```python
from build123d import *

# Parameters (mm, degrees)
BOSS_EXTRUDE1_DEPTH = 18
SKETCH6_W           = 70
SKETCH6_H           = 36
SKETCH6_R           = 2.5
BOSS_EXTRUDE2_DEPTH = 5
SKETCH7_R           = 10
CUT_EXTRUDE1_DEPTH  = 19
SKETCH8_R           = 14.2875
CUT_EXTRUDE2_DEPTH  = 6.35
CHAMFER1_SIZE       = 0.5
BOSS_EXTRUDE3_DEPTH = 6.35
BOSS_EXTRUDE4_DEPTH = 6.35


with BuildPart() as part:
    # Sketch3 → Boss-Extrude1 (new body)
    with BuildSketch(Plane.XY):
        with BuildLine():
            Line((-20, 0), (-20, -40))
            Line((-20, -40), (20, -40))
            Line((20, -40), (20, 0))
            ThreePointArc((20, 0), (0, 20), (-20, 0))
        make_face()
    extrude(amount=BOSS_EXTRUDE1_DEPTH)

    # Sketch6 → Boss-Extrude2 (add)
    with BuildSketch(Plane.XZ.offset(40)):
        Rectangle(SKETCH6_W, SKETCH6_H)
        with Locations((28, 0)):
            Circle(SKETCH6_R, mode=Mode.SUBTRACT)
        with Locations((-28, 0)):
            Circle(SKETCH6_R, mode=Mode.SUBTRACT)
    extrude(amount=BOSS_EXTRUDE2_DEPTH)

    # Sketch7 → Cut-Extrude1 (cut, through all)
    with BuildSketch(Plane(origin=(0, 0, 0), x_dir=(-1, 0, 0), z_dir=(0, 0, -1))):
        Circle(SKETCH7_R)
    extrude(amount=-CUT_EXTRUDE1_DEPTH, mode=Mode.SUBTRACT)

    # Sketch8 → Cut-Extrude2 (cut)
    with BuildSketch(Plane(origin=(0, 0, 0), x_dir=(-1, 0, 0), z_dir=(0, 0, -1))):
        Circle(SKETCH8_R)
    extrude(amount=-CUT_EXTRUDE2_DEPTH, mode=Mode.SUBTRACT)

    # Chamfer1
    chamfer1_edges = [part.edges().sort_by_distance(p)[0] for p in [
        (14.2875, 0, 0),
    ]]
    chamfer(chamfer1_edges, length=CHAMFER1_SIZE)

    # Sketch9 → Boss-Extrude3 (add)
    with BuildSketch(Plane(origin=(20, 0, 0), x_dir=(0, 0, -1), z_dir=(1, 0, 0))):
        Polygon((18, -40), (0, -10), (0, -40), align=None)
    boss_extrude3 = extrude(amount=-BOSS_EXTRUDE3_DEPTH)

    # Mirror1: Boss-Extrude3 across plane
    add(boss_extrude3.mirror(Plane(origin=(0, 0, 0), x_dir=(0, 0, 1), z_dir=(1, 0, 0))))

    # Sketch10 → Boss-Extrude4 (add)
    with BuildSketch(Plane.XY.offset(18)):
        Polygon((-20, -10), (-35, -40), (-20, -40), align=None)
        Polygon((20, -10), (20, -40), (35, -40), align=None)
    extrude(amount=-BOSS_EXTRUDE4_DEPTH)


solid = part.part
```
Geometry: final body of the model. Coordinates: model frame, mm. A direction names the side the tool comes from. Give positions to 0.01 mm unless a question says otherwise; leave off trailing zeros. Loops run counter-clockwise (first coordinate to the right, second up) from the corner with the lowest first, then second, coordinate; pieces in that order, holes last. Notation, with made-up numbers: (25, -18) -> (82, -18) arc R21 ccw to (82, -10) -> close; hole circle Ø10 at (-33, 12). An arc over 180 degrees is marked (long way). Return JSON: item names as keys, results as strings.
Item 1: Pin query (flat end, axial travel): P1, Ø6, axis at x = -28, z = 0, coming from the +Y side; P2, Ø3, axis at y = -25.5, z = 5, coming from the -X side; P3, Ø11, axis at y = -24, z = 1.5, coming from the +X side. Return the tip coordinate at first contact, or that it passes through.
Filled in:
{"P1": "y = -40", "P2": "x = -20", "P3": "x = 20"}
Item 2: Section B-B, the plane z = 10. Output: boundary loops of the cut face in (x, y), plus the area to 3 significant figures.
Filled in:
{"outline": "(-35, -45) -> (35, -45) -> (35, -40) -> (20, -40) -> (20, 0) arc R20 ccw to (-20, 0) -> (-20, -40) -> (-35, -40) -> close; hole circle Ø20 at (0, 0)", "area": "2,260 mm^2"}
Item 3: Section A-A, the plane x = 28. Output: boundary loops of the cut face in (y, z).
Filled in:
{"outline": "(-45, -18) -> (-40, -18) -> (-40, -2.5) -> (-45, -2.5) -> close; (-45, 2.5) -> (-40, 2.5) -> (-40, 11.65) -> (-26, 11.65) -> (-26, 18) -> (-45, 18) -> close"}
Item 4: Line query: line 1 (Y direction, x = 0, z = 9); line 2 (Y direction, x = 0, z = 1); line 3 (Y direction, x = 4, z = -5). Output: solid intervals per line, ascending.
Filled in:
{"line 1": "-45 to -10, 10 to 20", "line 2": "-45 to -14.29, 14.29 to 20", "line 3": "-45 to -40"}
Item 5: Section D-D, the plane x = -29.5. Output: boundary loops of the cut face in (y, z).
Filled in:
{"outline": "(-45, -18) -> (-40, -18) -> (-40, -2) -> (-45, -2) -> close; (-45, 2) -> (-40, 2) -> (-40, 11.65) -> (-29, 11.65) -> (-29, 18) -> (-45, 18) -> close"}
Item 6: Mould query, pull axis Y, two halves, no side actions, for faces 1 (the flat face through (27, -40, -3)), 2 (the cylindrical face through (14.274, 0.628, 3.384)), 3 (the flat face through (10, -3, 6.35)), 4 (the flat face through (-13.65, -31, -5)). Classes: released by +Y, released by -Y, zero draft, split by the parting line, or undercut.
Filled in:
{"face 1": "released by +Y", "face 2": "undercut", "face 3": "undercut", "face 4": "zero draft"}
Item 7: Section C-C, the plane y = -21. Output: boundary loops of the cut face in (x, z).
Filled in:
{"outline": "(-25.5, 11.65) -> (-20, 11.65) -> (-20, -6.6) -> (-13.65, -6.6) -> (-13.65, 0) -> (13.65, 0) -> (13.65, -6.6) -> (20, -6.6) -> (20, 11.65) -> (25.5, 11.65) -> (25.5, 18) -> (-25.5, 18) -> close"}
Item 8: Access query for faces 5 (the flat face through (13.65, -31, -5)), 6 (the flat face through (-20, -20, 0)), 7 (the flat face through (20, -20, 0)). Directions: +Z, -Z, +X, -X, +Y, -Y. A direction counts if a zero-diameter tool reaches every point of the face in a straight line with its end or side. Return the directions, or none.
Filled in:
{"face 5": "-Z, +Y", "face 6": "-Z, -X, +Y", "face 7": "-Z, +X, +Y"}
